Could you check a few things on this model? Use its own coordinates, in mm. A direction names the side the tool comes from. Round coordinates to 2 decimals unless told otherwise and drop trailing zeros. Loops run counter-clockwise (first coordinate to the right, second up) from the corner with the lowest first, then second, coordinate; pieces in that order, holes last. Notation, with made-up numbers: (2, 40) -> (10, 40) arc R10 cw to (10, 48) -> close; hole circle Ø5 at (21, 66). An arc over 180 degrees is marked (long way). One line per item, written item: value.
```python
from build123d import *

# Parameters (mm, degrees)
F3_R      = 2.5
F4_DEPTH  = 6
F6_DEPTH  = 1
F7_COUNT  = 3
F9_R      = 1.5
F10_DEPTH = 25


with BuildPart() as f1:
    # F0 (on Front) → F1 (revolve)
    with BuildSketch(Plane.XZ):
        with BuildLine():
            Line((-24, 12.5), (-24, 10))
            Line((-24, 10), (-6, 10))
            ThreePointArc((-6, 10), (-3.8786796564, 9.1213203436), (-3, 7))
            Line((-3, 7), (-3, 6.6722166417))
            ThreePointArc((-3, 6.6722166417), (-2.3420201433, 5.7325240209), (-1.2339555569, 6.029429032))
            Line((-1.2339555569, 6.029429032), (0, 7.5))
            Line((0, 7.5), (0, 11))
            Line((0, 11), (-22, 11))
            Line((-22, 11), (-22, 12.5))
            Line((-22, 12.5), (-24, 12.5))
        make_face()
    revolve(axis=Axis((0, 0, 0), (1, 0, 0)))



with BuildPart() as f4:
    # F3 (on offset) → F4 (new body)
    with BuildSketch(Plane.YZ.offset(-11)):
        Circle(F3_R)
    extrude(amount=F4_DEPTH)


with BuildPart() as f1_1:
    add(f1.part)

    add(f4.part)  # F6 merges F4
    # F5 (on face) → F6 (join)
    with BuildSketch(Plane(origin=(-11, 0, 0), x_dir=(0, -1, 0), z_dir=(-1, 0, 0))):
        with BuildLine():
            Line((0.75, 2.3848480035), (0.75, 9.9718353376))
            ThreePointArc((0.75, 9.9718353376), (0, 10), (-0.75, 9.9718353376))
            Line((-0.75, 9.9718353376), (-0.75, 2.3848480035))
            ThreePointArc((-0.75, 2.3848480035), (0, 2.5), (0.75, 2.3848480035))
        make_face()
    extrude(amount=-F6_DEPTH)


with BuildPart() as f7_1:
    # F7: instance of F1
    add(f1_1.part.rotate(Axis((-11, 0, 0), (1, 0, 0)), 1 * 360 / F7_COUNT))


with BuildPart() as f7_2:
    # F7: instance of F1
    add(f1_1.part.rotate(Axis((-11, 0, 0), (1, 0, 0)), 2 * 360 / F7_COUNT))


with BuildPart() as f1_2:
    add(f1_1.part)

    # F8: union F7_2, F7_1
    add(f7_2.part)
    add(f7_1.part)

    # F9 (on face) → F10 (cut)
    with BuildSketch(Plane(origin=(-11, 0, 0), x_dir=(0, -1, 0), z_dir=(-1, 0, 0))):
        Circle(F9_R)
    extrude(amount=-F10_DEPTH, mode=Mode.SUBTRACT)


solid = f1_2.part
```
Item 1: Will these pins go through, and if not, where does the flat tip stop? pin 1 Ø5 at (x, z) = (-11, 4) entering from +Y; pin 2 Ø10 at (x, z) = (-18.5, -6) entering from -Y; pin 3 Ø10 at (x, z) = (-21, 8.5) entering from -Y; pin 4 Ø2.5 at (y, z) = (0, 0) entering from -X.
Output:
pin 1: stops at y = 10.9
pin 2: stops at y = -12.26
pin 3: stops at y = -11.97
pin 4: passes through
Item 2: I need wall thicknesses on line 1 (Y direction, x = -13.5, z = 0); line 2 (Y direction, x = -10.5, z = -1.25); line 3 (X direction, y = 4, z = -11.5). Which ranges of each line are inside material? Lowest first, please. Write a range as from..to.
Output:
line 1: y = -11..-10, 10..11
line 2: y = -10.93..-9.92, -3.67..-0.83, 0.83..3.67, 9.92..10.93
line 3: x = -24..-22
Item 3: If we section it at D-D on x = -15: List the corners of the cut face in (y, z) for me.
Output:
outline: circle Ø22 at (0, 0); hole circle Ø20 at (0, 0)
Item 4: For faces 1 (the face through (-8.04, -0.54, -2.44)), 2 (the face through (-10, 5, -3)), 3 (the face through (-11, -1.1, -1.4)), which set-ups out of +Z, -Z, +X, -X, +Y, -Y let a thin tool reach every point of the face, with its end or its side?
Output:
face 1: +X
face 2: none
face 3: -X
Item 5: If we mould it in two halves opening along Z, with no side actions, what happens to faces 4 (the face through (-10.507, -4.93, -3.712)), 5 (the face through (-24, -10.2, -0.1)), 6 (the face through (-23.014, -3.755, 11.923))? For each: released by +Z, released by -Z, zero draft, split by the parting line, or undercut.
Output:
face 4: undercut
face 5: zero draft
face 6: split by the parting line
Item 6: If we section it at C-C on z = 0: List the corners of the cut face in (x, y) for me.
Output:
outline: (-24, -12.5) -> (-22, -12.5) -> (-22, -11) -> (0, -11) -> (0, -7.5) -> (-1.23, -6.03) arc R1 ccw to (-3, -6.67) -> (-3, -7) arc R3 cw to (-6, -10) -> (-24, -10) -> close; (-24, 10) -> (-6, 10) arc R3 cw to (-3, 7) -> (-3, 6.67) arc R1 ccw to (-1.23, 6.03) -> (0, 7.5) -> (0, 11) -> (-22, 11) -> (-22, 12.5) -> (-24, 12.5) -> close; (-11, -2.5) -> (-5, -2.5) -> (-5, -1.5) -> (-11, -1.5) -> close; (-11, 1.5) -> (-5, 1.5) -> (-5, 2.5) -> (-11, 2.5) -> close
Item 7: If we section it at B-B on x = -7.5: List the corners of the cut face in (y, z) for me, plus the area to 3 significant figures.
Output:
outline: circle Ø22 at (0, 0); circle Ø5 at (0, 0); hole circle Ø20 at (0, 0); hole circle Ø3 at (0, 0)
area: 78.5 mm²
Item 8: If we section it at A-A on y = 0: Count the separate pieces of the cut face and the enclosed holes in it, plus the area to 3 significant figures.
Output:
separate pieces: 3
enclosed holes: 0
area: 100 mm²
